```python
from build123d import *

# Parameters (mm, degrees)
SMUSSO1_SIZE                  = 0.5
SMUSSO2_SIZE                  = 1
TAGLIO_ESTRUSIONE1_DEPTH      = 16
TAGLIO_ESTRUSIONE1_DEPTH_BACK = 16
SCHIZZO2_W                    = 130
SCHIZZO2_H                    = 18
RACCORDO1_R                   = 0.5
RACCORDO2_R                   = 16
RACCORDO3_R                   = 2
SCHIZZO3_W                    = 4
SCHIZZO3_H                    = 18.361474643
SCHIZZO6_R                    = 52.5
ESTRUSIONE_ESTRUSIONE1_DEPTH  = 70
TAGLIO_ESTRUSIONE2_DEPTH      = 14
TAGLIO_ESTRUSIONE2_DEPTH_BACK = 14
SCHIZZO4_W                    = 155
SCHIZZO4_H                    = 16
RACCORDO4_R                   = 14
RACCORDO5_R                   = 0.5
ESTRUSIONE_ESTRUSIONE2_START  = 13
SCHIZZO7_R                    = 47.5
ESTRUSIONE_ESTRUSIONE2_DEPTH  = 13
SMUSSO3_SIZE                  = 1


with BuildPart() as part:
    # Schizzo1 → Rivoluzione1 (revolve)
    with BuildSketch(Plane.XY, mode=Mode.PRIVATE) as rivoluzione1_sk:
        Polygon((0, 0), (0, 52.5), (259, 52.5), (259, 55), (554, 55), (554, 65), (572.7, 65), (572.7, 47.5), (628.3, 47.5), (628.3, 0), align=None)
    revolve(rivoluzione1_sk.sketch.rotate(Axis((-197.2323049, 0, 0), (1, 0, 0)), 90), axis=Axis((-197.2323049, 0, 0), (1, 0, 0)))

    # Smusso1
    smusso1_edges = [part.edges().sort_by_distance(p)[0] for p in [
        (259, 0, -52.5),
    ]]
    chamfer(smusso1_edges, length=SMUSSO1_SIZE)

    # Smusso2
    smusso2_edges = [part.edges().sort_by_distance(p)[0] for p in [
        (572.7, 0, -47.5),
    ]]
    chamfer(smusso2_edges, length=SMUSSO2_SIZE)

    # Schizzo2 → Taglio-Estrusione1 (cut, two sides: drawn at the far end of the back side and taken through both)
    with BuildSketch(Plane.XY.offset(-TAGLIO_ESTRUSIONE1_DEPTH_BACK)):
        with Locations((484, 53)):
            Rectangle(SCHIZZO2_W, SCHIZZO2_H)
    extrude(amount=TAGLIO_ESTRUSIONE1_DEPTH + TAGLIO_ESTRUSIONE1_DEPTH_BACK, mode=Mode.SUBTRACT)

    # Raccordo1
    raccordo1_edges = [part.edges().sort_by_distance(p)[0] for p in [
        (549, 44, 0),
        (484, 44, 16),
        (419, 44, 0),
        (484, 44, -16),
    ]]
    fillet(raccordo1_edges, radius=RACCORDO1_R)

    # Raccordo2
    # the kernel refuses this fillet: 16 mm, written as the material it adds along each edge
    with BuildSketch(Plane(origin=(533, 44, 0), x_dir=(1, 0, 0), z_dir=(0, 0, -1))) as raccordo2_piece_1:
        with BuildLine():
            CenterArc((15.5, -0.5), 0.5, 0, 90)
            Line((16, -0.5), (16, 0))
            Line((16, 0), (15.5, 0))
        make_face()
    revolve(axis=Axis((533, 44, 0), (0, -1, 0)), revolution_arc=90)
    with BuildSketch(Plane(origin=(435, 44, 0), x_dir=(-1, 0, 0), z_dir=(0, 0, 1))) as raccordo2_piece_2:
        with BuildLine():
            CenterArc((15.5, -0.5), 0.5, 0, 90)
            Line((16, -0.5), (16, 0))
            Line((16, 0), (15.5, 0))
        make_face()
    revolve(axis=Axis((435, 44, 0), (0, -1, 0)), revolution_arc=90)
    with BuildSketch(Plane(origin=(435, 44, 0), x_dir=(0, 0, 1), z_dir=(1, 0, 0))) as raccordo2_piece_3:
        with BuildLine():
            CenterArc((15.5, -0.5), 0.5, 0, 90)
            Line((16, -0.5), (16, 0))
            Line((16, 0), (15.5, 0))
        make_face()
    revolve(axis=Axis((435, 44, 0), (0, -1, 0)), revolution_arc=90)
    with BuildSketch(Plane(origin=(533, 44, 0), x_dir=(0, 0, -1), z_dir=(-1, 0, 0))) as raccordo2_piece_4:
        with BuildLine():
            CenterArc((15.5, -0.5), 0.5, 0, 90)
            Line((16, -0.5), (16, 0))
            Line((16, 0), (15.5, 0))
        make_face()
    revolve(axis=Axis((533, 44, 0), (0, -1, 0)), revolution_arc=90)
    with BuildSketch(Plane(origin=(549, 92.621288468, -16), x_dir=(-1, 0, 0), z_dir=(0, -1, 0))) as raccordo2_piece_5_section:
        with BuildLine():
            CenterArc((RACCORDO2_R, -RACCORDO2_R), RACCORDO2_R, 90, 90)
            Line((0, -RACCORDO2_R), (0, 0))
            Line((0, 0), (RACCORDO2_R, 0))
        make_face()
    raccordo2_piece_5 = extrude(amount=48.621288468, mode=Mode.PRIVATE)
    raccordo2_piece_5 = raccordo2_piece_5 & Plane(origin=(545.534076623, 0, 0), x_dir=(0, 0, 1), z_dir=(1, 0, 0)) * Cylinder(55, 162, mode=Mode.PRIVATE)
    add(raccordo2_piece_5)
    with BuildSketch(Plane(origin=(419, 44, 16), x_dir=(0, 0, -1), z_dir=(0, 1, 0))) as raccordo2_piece_6_section:
        with BuildLine():
            CenterArc((RACCORDO2_R, -RACCORDO2_R), RACCORDO2_R, 90, 90)
            Line((0, -RACCORDO2_R), (0, 0))
            Line((0, 0), (RACCORDO2_R, 0))
        make_face()
    raccordo2_piece_6 = extrude(amount=48.621288468, mode=Mode.PRIVATE)
    raccordo2_piece_6 = raccordo2_piece_6 & Plane(origin=(422.465920441, 0, 0), x_dir=(0, 0, 1), z_dir=(1, 0, 0)) * Cylinder(55, 162, mode=Mode.PRIVATE)
    add(raccordo2_piece_6)
    with BuildSketch(Plane(origin=(419, 44, -16), x_dir=(0, 0, 1), z_dir=(0, 1, 0))) as raccordo2_piece_7_section:
        with BuildLine():
            CenterArc((RACCORDO2_R, RACCORDO2_R), RACCORDO2_R, 180, 90)
            Line((0, RACCORDO2_R), (0, 0))
            Line((0, 0), (RACCORDO2_R, 0))
        make_face()
    raccordo2_piece_7 = extrude(amount=48.621288468, mode=Mode.PRIVATE)
    raccordo2_piece_7 = raccordo2_piece_7 & Plane(origin=(422.465924893, 0, 0), x_dir=(0, 0, 1), z_dir=(1, 0, 0)) * Cylinder(55, 162, mode=Mode.PRIVATE)
    add(raccordo2_piece_7)
    with BuildSketch(Plane(origin=(549, 92.621288468, 16), x_dir=(-1, 0, 0), z_dir=(0, -1, 0))) as raccordo2_piece_8_section:
        with BuildLine():
            CenterArc((RACCORDO2_R, RACCORDO2_R), RACCORDO2_R, 180, 90)
            Line((0, RACCORDO2_R), (0, 0))
            Line((0, 0), (RACCORDO2_R, 0))
        make_face()
    raccordo2_piece_8 = extrude(amount=48.621288468, mode=Mode.PRIVATE)
    raccordo2_piece_8 = raccordo2_piece_8 & Plane(origin=(545.534073929, 0, 0), x_dir=(0, 0, 1), z_dir=(1, 0, 0)) * Cylinder(55, 162, mode=Mode.PRIVATE)
    add(raccordo2_piece_8)

    # Raccordo3
    raccordo3_edges = [part.edges().sort_by_distance(p)[0] for p in [
        (554, 0, -55),
    ]]
    fillet(raccordo3_edges, radius=RACCORDO3_R)

    # Schizzo3 → Taglia-Rivoluzione1 (revolve, cut)
    with BuildSketch(Plane.XY, mode=Mode.PRIVATE) as taglia_rivoluzione1_sk:
        with Locations((412, 62.180737322)):
            Rectangle(SCHIZZO3_W, SCHIZZO3_H)
    revolve(taglia_rivoluzione1_sk.sketch.rotate(Axis((-65.307499475, 0, 0), (1, 0, 0)), 90), axis=Axis((-65.307499475, 0, 0), (1, 0, 0)), mode=Mode.SUBTRACT)

    # Schizzo6 → Estrusione-Estrusione1 (add)
    with BuildSketch(Plane.ZY):
        Circle(SCHIZZO6_R)
    extrude(amount=ESTRUSIONE_ESTRUSIONE1_DEPTH)

    # Schizzo4 → Taglio-Estrusione2 (cut, two sides: drawn at the far end of the back side and taken through both)
    with BuildSketch(Plane.XY.offset(-TAGLIO_ESTRUSIONE2_DEPTH_BACK)):
        with Locations((57.5, 50.5)):
            Rectangle(SCHIZZO4_W, SCHIZZO4_H)
    extrude(amount=TAGLIO_ESTRUSIONE2_DEPTH + TAGLIO_ESTRUSIONE2_DEPTH_BACK, mode=Mode.SUBTRACT)

    # Raccordo4
    # the kernel refuses this fillet: 14 mm, written as the material it adds along each edge
    with BuildSketch(Plane(origin=(135, 85.598913032, 14), x_dir=(-1, 0, 0), z_dir=(0, -1, 0))) as raccordo4_piece_1_section:
        with BuildLine():
            CenterArc((RACCORDO4_R, RACCORDO4_R), RACCORDO4_R, 180, 90)
            Line((0, RACCORDO4_R), (0, 0))
            Line((0, 0), (RACCORDO4_R, 0))
        make_face()
    raccordo4_piece_1 = extrude(amount=78.098913032, mode=Mode.PRIVATE)
    raccordo4_piece_1 = raccordo4_piece_1 & Plane(origin=(131.948408204, 0, 0), x_dir=(0, 0, 1), z_dir=(1, 0, 0)) * Cylinder(52.5, 213, mode=Mode.PRIVATE)
    add(raccordo4_piece_1)
    with BuildSketch(Plane(origin=(135, 85.598913032, -14), x_dir=(0, 0, 1), z_dir=(0, -1, 0))) as raccordo4_piece_2_section:
        with BuildLine():
            CenterArc((RACCORDO4_R, RACCORDO4_R), RACCORDO4_R, 180, 90)
            Line((0, RACCORDO4_R), (0, 0))
            Line((0, 0), (RACCORDO4_R, 0))
        make_face()
    raccordo4_piece_2 = extrude(amount=78.098913032, mode=Mode.PRIVATE)
    raccordo4_piece_2 = raccordo4_piece_2 & Plane(origin=(131.948403613, 0, 0), x_dir=(0, 0, 1), z_dir=(1, 0, 0)) * Cylinder(52.5, 213, mode=Mode.PRIVATE)
    add(raccordo4_piece_2)
    with BuildSketch(Plane(origin=(-20, 7.5, 14), x_dir=(0, 0, -1), z_dir=(0, 1, 0))) as raccordo4_piece_3_section:
        with BuildLine():
            CenterArc((RACCORDO4_R, -RACCORDO4_R), RACCORDO4_R, 90, 90)
            Line((0, -RACCORDO4_R), (0, 0))
            Line((0, 0), (RACCORDO4_R, 0))
        make_face()
    raccordo4_piece_3 = extrude(amount=78.098913032, mode=Mode.PRIVATE)
    raccordo4_piece_3 = raccordo4_piece_3 & Plane(origin=(-16.8304684, 0, 0), x_dir=(0, 0, 1), z_dir=(1, 0, 0)) * Cylinder(52.5, 213, mode=Mode.PRIVATE)
    add(raccordo4_piece_3)
    with BuildSketch(Plane(origin=(-20, 7.5, -14), x_dir=(0, 0, 1), z_dir=(0, 1, 0))) as raccordo4_piece_4_section:
        with BuildLine():
            CenterArc((RACCORDO4_R, RACCORDO4_R), RACCORDO4_R, 180, 90)
            Line((0, RACCORDO4_R), (0, 0))
            Line((0, 0), (RACCORDO4_R, 0))
        make_face()
    raccordo4_piece_4 = extrude(amount=78.098913032, mode=Mode.PRIVATE)
    raccordo4_piece_4 = raccordo4_piece_4 & Plane(origin=(-16.8304684, 0, 0), x_dir=(0, 0, 1), z_dir=(1, 0, 0)) * Cylinder(52.5, 213, mode=Mode.PRIVATE)
    add(raccordo4_piece_4)

    # Raccordo5
    raccordo5_edges = [part.edges().sort_by_distance(p)[0] for p in [
        (57.5, 42.5, 14),
        (57.5, 42.5, -14),
        (-20, 42.5, 0),
        (-20, 42.5, 0),
        (135, 42.5, 0),
        (135, 42.5, 0),
    ]]
    fillet(raccordo5_edges, radius=RACCORDO5_R)

    # Schizzo7 → Estrusione-Estrusione2 (add)
    with BuildSketch(Plane(origin=(628.3, 0, 0), x_dir=(0, 0, -1), z_dir=(1, 0, 0)).offset(ESTRUSIONE_ESTRUSIONE2_START)):
        with Locations(Location((0, 0, 0), (0, 0, 180))):
            Circle(SCHIZZO7_R)
    extrude(amount=-ESTRUSIONE_ESTRUSIONE2_DEPTH)

    # Smusso3
    smusso3_edges = [part.edges().sort_by_distance(p)[0] for p in [
        (-70, 0, -52.5),
        (641.3, 0, -47.5),
    ]]
    chamfer(smusso3_edges, length=SMUSSO3_SIZE)


solid = part.part
```
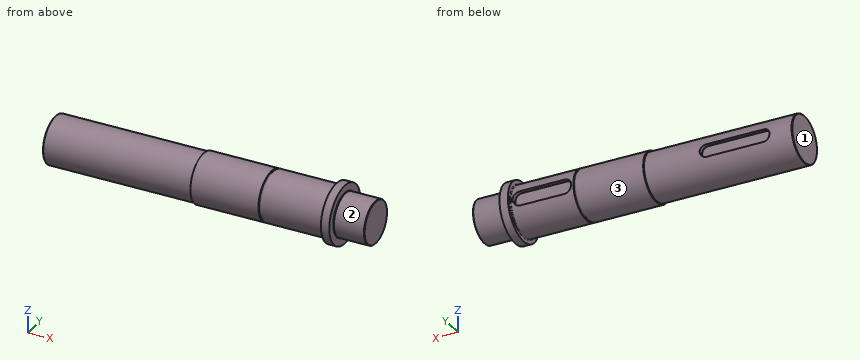
Source: CAD feature listing. Evaluate the final solid. Frame: model axes, mm. Face numbers are marked on the shaded views. A direction names the side the tool comes from. Round coordinates to 2 decimals unless told otherwise and drop trailing zeros. Order: outer loops, then holes, each group sorted by start corner. A loop starts at its lowest first (then second) coordinate and runs counter-clockwise, first axis right, second up. Notation, with made-up numbers: (33, 83.25) -> (61, 83.25) arc R23 cw to (61, 101.25) -> close; hole circle Ø4 at (17, 32.25). An arc over 180 degrees is marked (long way). One line per item, written item: value. Start each with the question number.
Q1. Pin query (flat end, axial travel): pin 1 (5 mm diameter, centred on x = 359, z = 39, fed in from +Y); pin 2 (1 mm diameter, centred on x = 405, y = -25.5, fed in from +Z); pin 3 (3 mm diameter, centred on x = 82, y = -37.5, fed in from -Z). Return the tip coordinate at first contact, or that it passes through.
Q2. Access query for the marked faces 1, 2 and 3. Directions: +Z, -Z, +X, -X, +Y, -Y. A direction counts if a zero-diameter tool reaches every point of the face in a straight line with its end or side. Return the directions, or none.
Q3. Material intervals for probe 1 along X at (y, z) = (-42, 33); probe 2 along X at (y, z) = (52, -12); probe 3 along Y at (x, z) = (376, 1.5), sorted ascending.
Q4. Section query B-B (x = 279.5). Return the cut outline in (y, z).
Findings below:
1. pin 1: y = 41.14
1. pin 2: z = 48.99
1. pin 3: z = -38.21
2. face 1: +Z, -Z, -X, +Y, -Y
2. face 2: +X
2. face 3: -X
3. probe 1: 259 to 410, 414 to 572.7
3. probe 2: 259 to 410, 414 to 424.42, 543.58 to 572.7
3. probe 3: -54.98 to 54.98
4. outline: circle Ø110 at (0, 0)
